Can you work these out from the drawing? Everything is in mm from the part's minimum corner. A direction names the side the tool comes from. Round coordinates to 2 decimals unless told otherwise and drop trailing zeros. Order: outer loops, then holes, each group sorted by start corner. A loop starts at its lowest first (then second) coordinate and runs counter-clockwise, first axis right, second up. Notation, with made-up numbers: (55, 44) -> (101, 44) arc R30 ccw to (101, 70) -> close; hole circle Ø6 at (80.5, 9). An arc over 180 degrees is marked (long way). One line per item, written item: value.
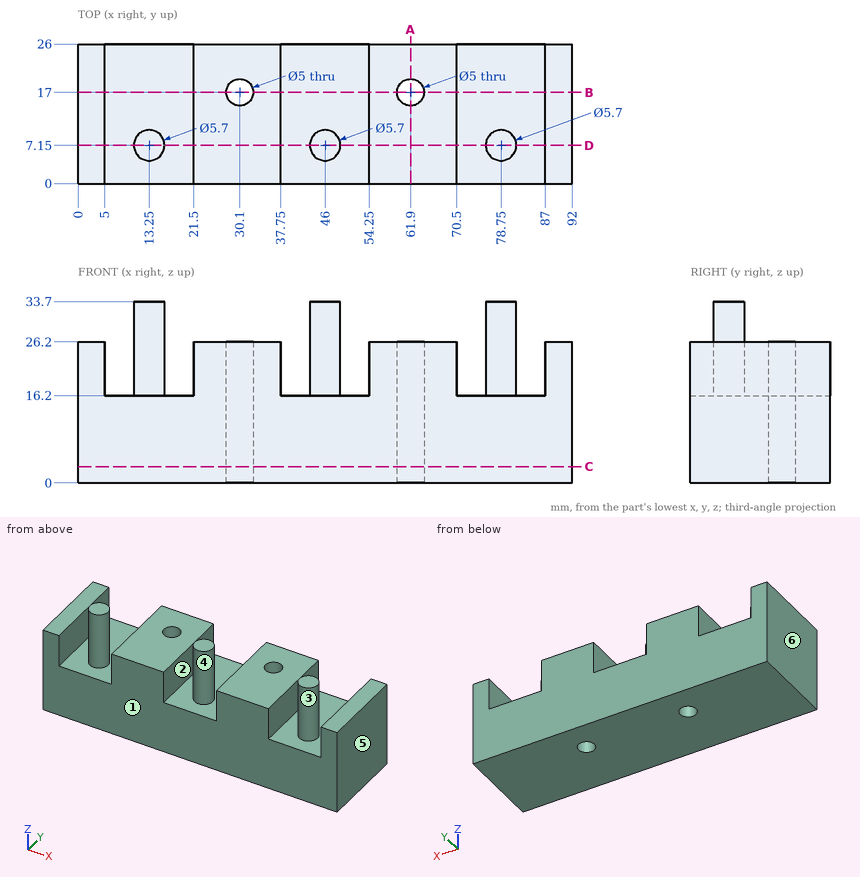
Q1. I want a section at B-B on y = 17. Write out the boundary of the cut face in (x, z).
Answers:
outline: (0, 0) -> (27.6, 0) -> (27.6, 26.2) -> (21.5, 26.2) -> (21.5, 16.2) -> (5, 16.2) -> (5, 26.2) -> (0, 26.2) -> close; (32.6, 0) -> (59.4, 0) -> (59.4, 26.2) -> (54.25, 26.2) -> (54.25, 16.2) -> (37.75, 16.2) -> (37.75, 26.2) -> (32.6, 26.2) -> close; (64.4, 0) -> (92, 0) -> (92, 26.2) -> (87, 26.2) -> (87, 16.2) -> (70.5, 16.2) -> (70.5, 26.2) -> (64.4, 26.2) -> close
Q2. I want a section at D-D on y = 7.15. Write out the boundary of the cut face in (x, z).
Answers:
outline: (0, 0) -> (92, 0) -> (92, 26.2) -> (87, 26.2) -> (87, 16.2) -> (81.6, 16.2) -> (81.6, 33.7) -> (75.9, 33.7) -> (75.9, 16.2) -> (70.5, 16.2) -> (70.5, 26.2) -> (54.25, 26.2) -> (54.25, 16.2) -> (48.85, 16.2) -> (48.85, 33.7) -> (43.15, 33.7) -> (43.15, 16.2) -> (37.75, 16.2) -> (37.75, 26.2) -> (21.5, 26.2) -> (21.5, 16.2) -> (16.1, 16.2) -> (16.1, 33.7) -> (10.4, 33.7) -> (10.4, 16.2) -> (5, 16.2) -> (5, 26.2) -> (0, 26.2) -> close
Q3. For P1, Ø8, axis at x = 32.5, y = 17.5, coming from the +Z side; P2, Ø4.5, axis at x = 30.1, y = 17, coming from the +Z side; P3, Ø8, axis at x = 74.5, z = 30, coming from the +Y side; P4, Ø1, axis at y = 4.5, z = 29.5, coming from the -X side, each with a flat end and sliding along its axis, tell me the tip position at first contact or that it passes through.
Answers:
P1: z = 26.2
P2: through
P3: y = 9.99
P4: x = 11.38
Q4. I need wall thicknesses on line 1 along Y through (x, z) = (61.9, 7.75); line 2 along Z through (x, y) = (48.5, 9); line 3 along Z through (x, y) = (63.5, 4.25). Which ranges of each line are inside material? Lowest first, please.
Answers:
line 1: 0 to 14.5, 19.5 to 26
line 2: 0 to 16.2
line 3: 0 to 26.2
Q5. I want a section at A-A on x = 61.9. Write out the boundary of the cut face in (y, z), then the cut area to 3 significant figures.
Answers:
outline: (0, 0) -> (14.5, 0) -> (14.5, 26.2) -> (0, 26.2) -> close; (19.5, 0) -> (26, 0) -> (26, 26.2) -> (19.5, 26.2) -> close
area: 550 mm2
Q6. If we mould it in two halves opening along X, with no side actions, what happens to the marked faces 4, 5 and 6? For each: pulls with the +X half, pulls with the -X half, needs draft (parallel to the pull), parting line crosses it, or undercut.
Answers:
face 4: undercut
face 5: pulls with the +X half
face 6: pulls with the -X half
Q7. I want a section at C-C on z = 3. Write out the boundary of the cut face in (x, y), then the cut area to 3 significant figures.
Answers:
outline: (0, 0) -> (92, 0) -> (92, 26) -> (0, 26) -> close; hole circle Ø5 at (30.1, 17); hole circle Ø5 at (61.9, 17)
area: 2,350 mm2
Q8. Which directions (+Z, -Z, +X, -X, +Y, -Y) give clear straight access to the entire face, cutting with the end or side of a thin tool? Please do the marked faces 1, 2 and 3.
Answers:
face 1: +Z, -Z, +X, -X, -Y
face 2: +Z, +Y, -Y
face 3: +Z
